```python
from build123d import *

# Parameters (mm, degrees)
BOSS_EXTRUDE2_DEPTH = 10.01387566
BOSS_EXTRUDE3_DEPTH = 12
SKETCH18_R          = 20
BOSS_EXTRUDE6_DEPTH = 40
SKETCH26_R          = 12.5
CUT_EXTRUDE2_DEPTH  = 40
CUT_EXTRUDE5_DEPTH  = 40
BOSS_EXTRUDE8_DEPTH = 5
BOSS_EXTRUDE9_DEPTH = 5


with BuildPart() as part:
    # Sketch1 → Boss-Extrude2 (new body)
    with BuildSketch(Plane(origin=(0, 0, 0), x_dir=(1, 0, 0), z_dir=(0, 1, 0))):
        with BuildLine():
            Line((-40, -25), (-40, -15))
            ThreePointArc((-40, -15), (-25, 0), (-40, 15))
            Line((-40, 15), (-40, 25))
            Line((-40, 25), (40.060765138, 20))
            Line((40.060765138, 20), (40.060765138, -20))
            Line((40.060765138, -20), (-40, -25))
        make_face()
    extrude(amount=BOSS_EXTRUDE2_DEPTH)

    # Sketch17 → Boss-Extrude3 (add)
    with BuildSketch(Plane(origin=(0, 0, 0), x_dir=(1, 0, 0), z_dir=(0, 1, 0))):
        with BuildLine():
            Line((-40, 25), (-40, 15))
            ThreePointArc((-40, 15), (-25, 0), (-40, -15))
            Line((-40, -15), (-40, -25))
            ThreePointArc((-40, -25), (-15, 0), (-40, 25))
        make_face()
    extrude(amount=BOSS_EXTRUDE3_DEPTH)

    # Sketch18 → Boss-Extrude6 (add)
    with BuildSketch(Plane(origin=(0, 0, 0), x_dir=(1, 0, 0), z_dir=(0, 1, 0))):
        with Locations(Location((39.84238711, 0, 0), (0, 0, 89.374380602))):
            Circle(SKETCH18_R)
    extrude(amount=BOSS_EXTRUDE6_DEPTH)

    # Sketch26 → Cut-Extrude2 (cut)
    with BuildSketch(Plane(origin=(0, 0, 0), x_dir=(1, 0, 0), z_dir=(0, 1, 0))):
        with Locations(Location((40.060765138, 0, 0), (0, 0, 270))):
            Circle(SKETCH26_R)
    extrude(amount=CUT_EXTRUDE2_DEPTH, mode=Mode.SUBTRACT)

    # Sketch27 → Cut-Extrude5 (cut)
    with BuildSketch(Plane(origin=(0, 0, 0), x_dir=(1, 0, 0), z_dir=(0, 1, 0))):
        with BuildLine():
            Line((55.060765138, 2.499608634), (52.235862007, 2.499608634))
            ThreePointArc((52.235862007, 2.499608634), (52.426066383, 1.256530998), (52.489684933, 0.00059613))
            ThreePointArc((52.489684933, 0.00059613), (52.426015439, -1.255840203), (52.235659276, -2.49940387))
            Line((52.235659276, -2.49940387), (55.060765138, -2.49940387))
            Line((55.060765138, -2.49940387), (55.060765138, 0.00059613))
            Line((55.060765138, 0.00059613), (55.060765138, 2.499608634))
        make_face()
    extrude(amount=CUT_EXTRUDE5_DEPTH, mode=Mode.SUBTRACT)

    # Sketch35 → Boss-Extrude8 (add)
    with BuildSketch(Plane.XY):
        Polygon((-15, 12), (-10, 12), (19.84238711, 32.5), (25.015627371, 36.053717903), (26.363273424, 32.5), (25.450319422, 10.01387566), (19.84238711, 10.01387566), (-15, 10.01387566), (-18.557885477, 10.01387566), (-18.07381102, 12), align=None)
    extrude(amount=BOSS_EXTRUDE8_DEPTH)

    # Sketch41 → Boss-Extrude9 (add)
    with BuildSketch(Plane.XY):
        Polygon((19.84238711, 32.5), (-10, 12), (-16.624555897, 12), (-16.624555897, 10.01387566), (29.789890708, 10.01387566), (27.477800575, 29.176181785), (25.597486792, 36.45342179), align=None)
    extrude(amount=-BOSS_EXTRUDE9_DEPTH)


solid = part.part
```
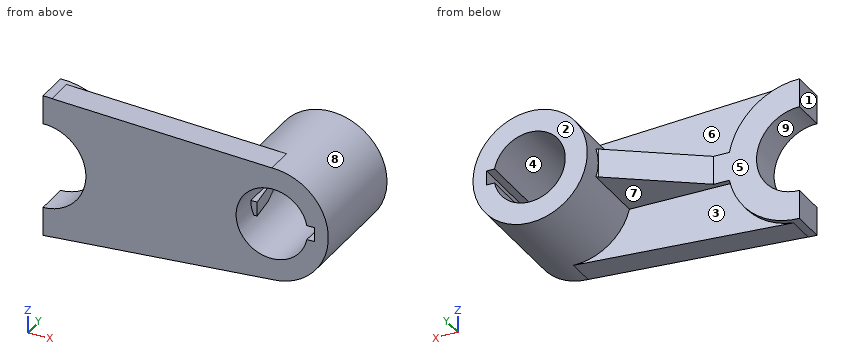
Geometry check sheet. Reference: the model listing, model coordinates, mm. Face numbers are marked on the shaded views. A direction names the side the tool comes from. Coordinates: 2 decimals unless noted, no trailing zeros. Order: outer loops, then holes, each group sorted by start corner. A loop starts at its lowest first (then second) coordinate and runs counter-clockwise, first axis right, second up.
Q1. Sectioned sample at C-C on x = -18. Record the cut outline in (y, z), and give its area (3 significant figures).
Reply:
outline: (0, -23.63) - (10.01, -23.63) - (10.01, -11.87) - (12, -11.87) - (12, 11.87) - (10.01, 11.87) - (10.01, 23.63) - (0, 23.63) - close
area: 520 mm2
Q2. Thickness scan on probe 1 along X at (y, z) = (23, -10); probe 2 along Y at (x, z) = (9, -16); probe 3 along Z at (x, y) = (46.5, 5.5). Record the ranges inside material, lowest first.
Reply:
probe 1: x = 22.52 to 32.56, 47.56 to 57.16
probe 2: y = 0 to 10.01
probe 3: z = -18.86 to -10.71, 10.71 to 18.86
Q3. Sectioned sample at D-D on z = -21. Record the cut outline in (x, y), and give its area (3 significant figures).
Reply:
outline: (-40, 0) - (24.05, 0) - (24.05, 10.01) - (-26.44, 10.01) - (-26.44, 12) - (-40, 12) - close
area: 668 mm2
Q4. Depth check by flat-ended pin: pin 1 Ø10 at (x, z) = (-24.5, -6.5) entering from +Y; pin 2 Ø3 at (x, y) = (54, 26.5) entering from -Z (3 decimals); pin 3 Ø1.5 at (x, y) = (12.5, 28.5) entering from -Z; pin 4 Ø5 at (x, y) = (49, 9) entering from -Z. Enter the tip coordinate at first touch or a pass-through.
Reply:
pin 1: stops at y = 12
pin 2: stops at z = -15.485
pin 3: passes through
pin 4: stops at z = -18.86
Q5. Draft check along X on the marked faces 1, 2, 3 and 4. Enter one of: released by +X, released by -X, zero draft, split by the parting line, or undercut.
Reply:
face 1: released by -X
face 2: zero draft
face 3: undercut
face 4: undercut
Q6. Sectioned sample at B-B on x = 34. Record the cut outline in (y, z).
Reply:
outline: (0, -20.38) - (10.01, -20.38) - (10.01, -19.13) - (40, -19.13) - (40, -10.93) - (0, -10.93) - close; (0, 10.93) - (40, 10.93) - (40, 19.13) - (10.01, 19.13) - (10.01, 20.38) - (0, 20.38) - close
Q7. Sectioned sample at A-A on y = 34.5. Record the cut outline in (x, z).
Reply:
outline: circle Ø40 at (39.84, 0); hole (52.31, -2.5) - (55.06, -2.5) - (55.06, 2.5) - (52.31, 2.5) arc R12.5 ccw (long way) to start
Q8. Tool access check on the marked faces 5, 6, 7, 8 and 9. Record the directions out of +Z, -Z, +X, -X, +Y, -Y that give a thin tool (end or side, any length) a straight path to the whole face; none if there is none.
Reply:
face 5: +Z, -Z, -X, +Y
face 6: +Z, +Y
face 7: -Z, +Y
face 8: +Y
face 9: -X, +Y, -Y
